from build123d import *

# Parameters (mm, degrees)
ESBO_O1_W                = 6
ESBO_O1_H                = 5.15
RESSALTO_EXTRUS_O1_DEPTH = 50
CORTE_EXTRUS_O5_START    = -2.575
CORTE_EXTRUS_O5_DEPTH    = 5.15
FILETE2_R                = 2
SKETCH1_W                = 100
SKETCH1_H                = 11
BOSS_EXTRUDE1_DEPTH      = 3
SKETCH2_W                = 100
SKETCH2_H                = 21
BOSS_EXTRUDE2_DEPTH      = 3
FILLET1_R                = 2
FILLET2_R                = 2
CUT_EXTRUDE1_START       = 2.825
CUT_EXTRUDE1_OUTLINE_R   = 1.5
CUT_EXTRUDE1_DEPTH       = 2.75
SKETCH6_W                = 5
SKETCH6_H                = 5.15
BOSS_EXTRUDE4_DEPTH      = 1.5
SKETCH8_R                = 1.5
CUT_EXTRUDE2_DEPTH       = 2.75
CHAMFER2_SIZE            = 1.25


# Read off the part's stored shape, not the designer's step: Corte-extrusão5, Cut-Extrude1
with BuildPart() as part:
    # Esboço1 → Ressalto-extrusão1 (new, symmetric)
    with BuildSketch(Plane(origin=(0, 0, 0), x_dir=(0, 0, -1), z_dir=(1, 0, 0))):
        with Locations((-3, 0)):
            Rectangle(ESBO_O1_W, ESBO_O1_H)
    extrude(amount=RESSALTO_EXTRUS_O1_DEPTH, both=True)

    # Corte-extrusão5 outline → Corte-extrusão5 (cut)
    with BuildSketch(Plane(origin=(0, 0, 0), x_dir=(1, 0, 0), z_dir=(0, 1, 0)).offset(CORTE_EXTRUS_O5_START)):
        Polygon((46, -6), (45, -1.2), (33, -6), align=None)
    extrude(amount=CORTE_EXTRUS_O5_DEPTH, mode=Mode.SUBTRACT)

    # Filete2
    filete2_edges = [part.edges().sort_by_distance(p)[0] for p in [
        (46, 0, 6),
    ]]
    fillet(filete2_edges, radius=FILETE2_R)

    # Sketch1 → Boss-Extrude1 (add)
    with BuildSketch(Plane(origin=(0, 2.575, 0), x_dir=(1, 0, 0), z_dir=(0, 1, 0))):
        with Locations((0, -5.5)):
            Rectangle(SKETCH1_W, SKETCH1_H)
    extrude(amount=BOSS_EXTRUDE1_DEPTH)

    # Sketch2 → Boss-Extrude2 (add)
    with BuildSketch(Plane.XZ.offset(2.575)):
        with Locations((0, 10.5)):
            Rectangle(SKETCH2_W, SKETCH2_H)
    extrude(amount=BOSS_EXTRUDE2_DEPTH)

    # Fillet1
    fillet1_edges = [part.edges().sort_by_distance(p)[0] for p in [
        (45, 0, 1.2),
    ]]
    fillet(fillet1_edges, radius=FILLET1_R)

    # Fillet2
    fillet2_edges = [part.edges().sort_by_distance(p)[0] for p in [
        (33, 0, 6),
    ]]
    fillet(fillet2_edges, radius=FILLET2_R)

    # Cut-Extrude1 outline → Cut-Extrude1 (cut)
    with BuildSketch(Plane(origin=(0, 0, 0), x_dir=(1, 0, 0), z_dir=(0, 1, 0)).offset(CUT_EXTRUDE1_START)):
        with Locations((-43.75, -5.5)):
            Circle(CUT_EXTRUDE1_OUTLINE_R)
        with Locations((43.75, -5.5)):
            Circle(CUT_EXTRUDE1_OUTLINE_R)
        with Locations((47, -2.25)):
            Circle(CUT_EXTRUDE1_OUTLINE_R)
        with Locations((47, -8.75)):
            Circle(CUT_EXTRUDE1_OUTLINE_R)
        with Locations((-47, -8.75)):
            Circle(CUT_EXTRUDE1_OUTLINE_R)
        with Locations((-47, -2.25)):
            Circle(CUT_EXTRUDE1_OUTLINE_R)
    extrude(amount=CUT_EXTRUDE1_DEPTH, mode=Mode.SUBTRACT)

    # Sketch6 → Boss-Extrude4 (add)
    with BuildSketch(Plane.ZY.offset(50)):
        with Locations((8.5, 0)):
            Rectangle(SKETCH6_W, SKETCH6_H)
    extrude(amount=-BOSS_EXTRUDE4_DEPTH)

    # Sketch8 → Cut-Extrude2 (cut)
    with BuildSketch(Plane.XZ.offset(5.575)):
        with Locations(Location((47, 8.75, 0), (0, 0, 90))):
            Circle(SKETCH8_R)
        with Locations(Location((43.75, 5.5, 0), (0, 0, 270))):
            Circle(SKETCH8_R)
        with Locations(Location((47, 2.25, 0), (0, 0, 270))):
            Circle(SKETCH8_R)
        with Locations(Location((-47, 8.75, 0), (0, 0, 270))):
            Circle(SKETCH8_R)
        with Locations(Location((-43.75, 5.5, 0), (0, 0, 90))):
            Circle(SKETCH8_R)
        with Locations(Location((-47, 2.25, 0), (0, 0, 90))):
            Circle(SKETCH8_R)
    extrude(amount=-CUT_EXTRUDE2_DEPTH, mode=Mode.SUBTRACT)

    # Chamfer2
    chamfer2_edges = [part.edges().sort_by_distance(p)[0] for p in [
        (50, 2.575, 8.5),
        (50, 0, 6),
    ]]
    chamfer(chamfer2_edges, length=CHAMFER2_SIZE)


solid = part.part
Work out the finished part from the listing and answer in its coordinate system (mm). A direction names the side the tool comes from. Round coordinates to 2 decimals unless told otherwise and drop trailing zeros. Loops run counter-clockwise (first coordinate to the right, second up) from the corner with the lowest first, then second, coordinate; pieces in that order, holes last. Notation, with made-up numbers: (81, 36) - (104, 36) arc R18 ccw to (104, 60) - close; hole circle Ø1 at (14.5, -27). An arc over 180 degrees is marked (long way). Use one line per item in the form item = value. Start each with the question number.
(1) Find section D-D on x = -11. Determine the outline of the cut face in (y, z) (3 decimals), and give its area (3 significant figures).
(2) Find section A-A on x = -43.75. Determine the outline of the cut face in (y, z) (3 decimals), and give its area (3 significant figures).
(3) Find section B-B on y = -4.5. Determine the outline of the cut face in (x, z), and give its area (3 significant figures).
(4) Consider line 1 (X direction, y = -3.5, z = 5.5); line 2 (Z direction, x = -47, y = 4.35); line 3 (X direction, y = -3.4, z = 2.25). Determine where each line is inside the solid, lowest interval first.
(5) Determine the mould class of faces 5 (the face through (45.5, 4.2, 2.2)), 6 (the face through (-1, -2.575, 14)), 7 (the face through (47, -2.825, 9)), 8 (the face through (44, 0, 2)) for opening direction Y: +Y half, -Y half, draft (parallel to the pull), parting line (faces both ways), or undercut.
(6) Find section C-C on z = 8.75. Determine the outline of the cut face in (x, y) (3 decimals), and give its area (3 significant figures).
(7) Which of the six approach directions +Z, -Z, +X, -X, +Y, -Y give full straight-line access (tool end or side, diameter ignored) to faces 1 (the face through (-47, 2.825, 9)), 2 (the face through (-48.464, -4.219, 9.075)), 3 (the face through (-7, 0, 6)), 4 (the face through (0, 4, 11))?
(8) Flat-ended cylindrical pins translate along their axes: P1, Ø1.5, axis at x = 44, z = 6, coming from the +Y side (3 decimals); P2, Ø2.5, axis at x = -43.75, z = 5.5, coming from the -Y side (3 decimals); P3, Ø5, axis at x = -32.5, y = 3.5, coming from the +Z side. Find the tip coordinate at first contact, or state that the pin passes through.
Answer list:
q1.outline = (-5.575, 0) - (5.575, 0) - (5.575, 11) - (2.575, 11) - (2.575, 6) - (-2.575, 6) - (-2.575, 21) - (-5.575, 21) - close
q1.area = 127 mm^2
q2.outline = (-5.575, 0) - (5.575, 0) - (5.575, 4) - (2.825, 4) - (2.825, 7) - (5.575, 7) - (5.575, 11) - (2.575, 11) - (2.575, 6) - (-2.575, 6) - (-2.575, 21) - (-5.575, 21) - (-5.575, 7) - (-2.825, 7) - (-2.825, 4) - (-5.575, 4) - close
q2.area = 110 mm^2
q3.outline = (-50, 0) - (50, 0) - (50, 21) - (-50, 21) - close; hole circle Ø3 at (-47, 2.25); hole circle Ø3 at (-47, 8.75); hole circle Ø3 at (-43.75, 5.5); hole circle Ø3 at (43.75, 5.5); hole circle Ø3 at (47, 2.25); hole circle Ø3 at (47, 8.75)
q3.area = 2,060 mm^2
q4.line_1 = -50 to -45.25, -42.25 to 42.25, 45.25 to 50
q4.line_2 = 0 to 0.75, 3.75 to 7.25, 10.25 to 11
q4.line_3 = -50 to -48.5, -45.5 to 45.5, 48.5 to 50
q5.face_5 = draft
q5.face_6 = undercut
q5.face_7 = -Y half
q5.face_8 = undercut
q6.outline = (-50, -5.575) - (-48.5, -5.575) - (-48.5, -2.825) - (-45.5, -2.825) - (-45.5, -5.575) - (45.5, -5.575) - (45.5, -2.825) - (48.5, -2.825) - (48.5, -5.575) - (50, -5.575) - (50, -2.575) - (-48.5, -2.575) - (-48.5, 2.575) - (48.75, 2.575) - (50, 3.825) - (50, 5.575) - (48.5, 5.575) - (48.5, 2.825) - (45.5, 2.825) - (45.5, 5.575) - (-45.5, 5.575) - (-45.5, 2.825) - (-48.5, 2.825) - (-48.5, 5.575) - (-50, 5.575) - close
q6.area = 574 mm^2
q7.face_1 = +Y
q7.face_2 = -Y
q7.face_3 = +Z, +X
q7.face_4 = +Z, +X, -X, +Y
q8.P1 = 2.825
q8.P2 = -2.825
q8.P3 = 11
